Geometry check sheet. Reference: drawing and pictorial views, mm from the part's lowest x, y, z. Give positions to 0.01 mm unless a question says otherwise; leave off trailing zeros. Write each loop counter-clockwise with the first axis right and the second up, starting at its lowest first coordinate (ties: lowest second). Pieces come first, ordered by that corner, then holes. Notation, with made-up numbers: (6.25, -39.75) -> (52.25, -39.75) arc R19 ccw to (52.25, -34.75) -> close; hole circle Ø3 at (15, 67). An arc over 180 degrees is marked (long way). Use a Markdown table: item, result. Add a question column.
1. Scan lines: probe 1 along Z at (x, y) = (115, 20.75); probe 2 along X at (y, z) = (17.5, 32.5); probe 3 along Z at (x, y) = (120, 9.75) (1 decimal). Record each from-to range of solid material in increasing order. Write a range as [from, to].
2. Gauge pin test, flat end, axial feed: P1, Ø6.5, axis at x = 115.32, z = 32.68, coming from the +Y side. Record the tip position at first contact, or that the pin passes through.
3. Release check for a two-part mould opening along Z. For the marked faces 1, 2, 3 and 4 record: released by +Z, released by -Z, zero draft, split by the parting line, or undercut.
4. Cross-section at A-A (z = 30.5). Enter the section's corners in (x, y) (1 decimal).
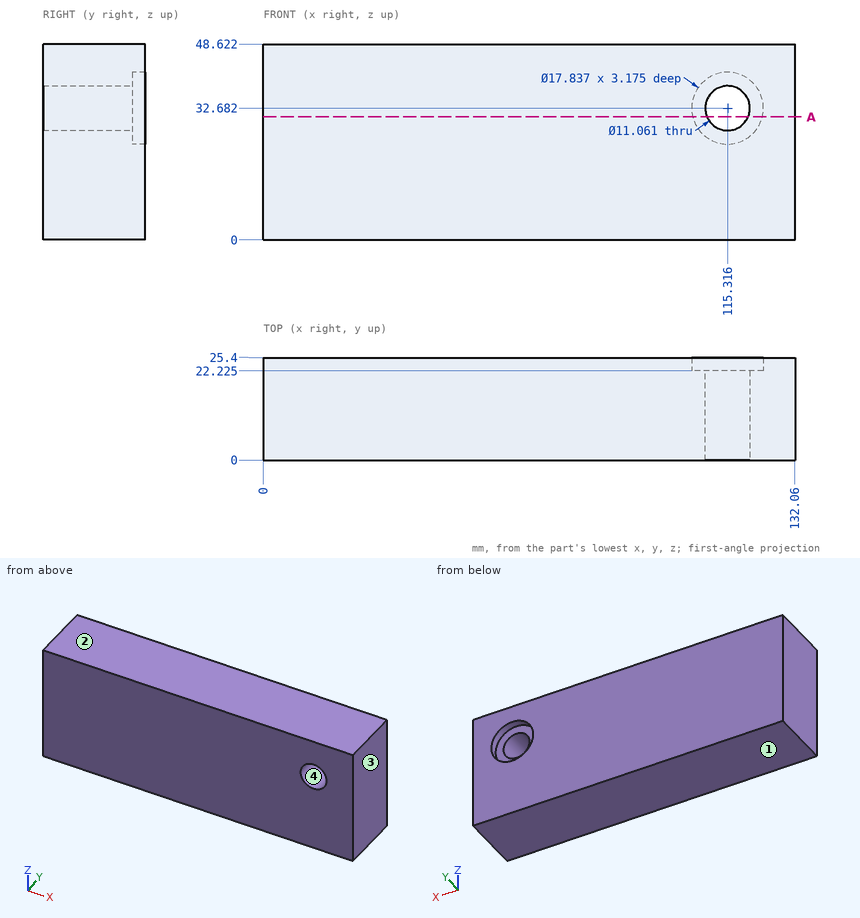
Worked answers:
| question | item | result |
|---|---|---|
| 1 | probe 1 | z = [0, 27.16], [38.2, 48.62] |
| 1 | probe 2 | x = [0, 109.79], [120.84, 132.06] |
| 1 | probe 3 | z = [0, 29.7], [35.6, 48.6] |
| 2 | P1 | passes through |
| 3 | face 1 | released by -Z |
| 3 | face 2 | released by +Z |
| 3 | face 3 | zero draft |
| 3 | face 4 | undercut |
| 4 | outline | (0, 0) -> (110.2, 0) -> (110.2, 22.2) -> (106.7, 22.2) -> (106.7, 25.4) -> (0, 25.4) -> close; (120.4, 0) -> (132.1, 0) -> (132.1, 25.4) -> (124, 25.4) -> (124, 22.2) -> (120.4, 22.2) -> close |
